from build123d import *

# Parameters (mm, degrees)
SKETCH1_R           = 25
BOSS_EXTRUDE1_DEPTH = 3
SKETCH2_R           = 1.75
CUT_EXTRUDE1_DEPTH  = 3
CIRPATTERN1_COUNT   = 8


with BuildPart() as part:
    # Sketch1 → Boss-Extrude1 (new body)
    with BuildSketch(Plane.XY):
        Circle(SKETCH1_R)
    extrude(amount=BOSS_EXTRUDE1_DEPTH)

    # Sketch2 → Cut-Extrude1 (cut)
    with BuildSketch(Plane.XY.offset(3)):
        with Locations((0, 20)):
            Circle(SKETCH2_R)
    cut_extrude1 = extrude(amount=-CUT_EXTRUDE1_DEPTH, mode=Mode.SUBTRACT)

    # CirPattern1: Cut-Extrude1 ×8 about axis
    cirpattern1_axis = Axis((0, 0, 0), (0, 0, 1))
    for i in range(1, CIRPATTERN1_COUNT):
        add(cut_extrude1.rotate(cirpattern1_axis, i * 360 / CIRPATTERN1_COUNT), mode=Mode.SUBTRACT)


solid = part.part
Model file for the job. Use its own axes, mm. Give positions to 0.01 mm unless a question says otherwise; leave off trailing zeros. Loops run counter-clockwise (first coordinate to the right, second up) from the corner with the lowest first, then second, coordinate; pieces in that order, holes last. Notation, with made-up numbers: (-18.75, 18.25) -> (-0.75, 18.25) arc R30 cw to (-0.75, 51.25) -> close; hole circle Ø11 at (86.25, 6.5). An arc over 180 degrees is marked (long way). Use a Markdown table: item, result. Add a question column.
(1) Wall check: line 1 along Y through (x, z) = (0, 2.2); line 2 along X through (y, z) = (-13, 0.1); line 3 along Y through (x, z) = (15, 0.35). Give the ranges that are in metal, low to high.
(2) Slice it at D-D on z = 0.8. Give the number of separate pieces and of enclosed holes in the cut face, and give its area (3 significant figures).
(3) Slice it at C-C on y = 0. List the corners of the cut face in (x, z).
(4) Mould opens along X. For faces 1 (the cylindrical face through (23.846, 7.509, 1.479)), 2 (the flat face through (0, 0, 3)), 3 (the cylindrical face through (12.525, -14.811, 1.521)) say: +X half, -X half, draft (parallel to the pull), parting line (faces both ways), or undercut.
(5) Drop flat-ended pins along their axis: pin 1 Ø3 at (x, y) = (14.14, 14.14) entering from +Z; pin 2 Ø1 at (y, z) = (-16.5, 2) entering from +X; pin 3 Ø1 at (x, y) = (15.5, -6) entering from -Z. Give the stop position or say it passes through.
(6) Slice it at A-A on y = 20. List the corners of the cut face in (x, z), and give its area (3 significant figures).
Filled sheet:
| question | item | result |
|---|---|---|
| 1 | line 1 | -25 to -21.75, -18.25 to 18.25, 21.75 to 25 |
| 1 | line 2 | -21.35 to -15.47, -12.82 to 12.82, 15.47 to 21.35 |
| 1 | line 3 | -20 to -15.67, -12.62 to 12.62, 15.67 to 20 |
| 2 | separate pieces | 1 |
| 2 | enclosed holes | 8 |
| 2 | area | 1,890 mm2 |
| 3 | outline | (-25, 0) -> (-21.75, 0) -> (-21.75, 3) -> (-25, 3) -> close; (-18.25, 0) -> (18.25, 0) -> (18.25, 3) -> (-18.25, 3) -> close; (21.75, 0) -> (25, 0) -> (25, 3) -> (21.75, 3) -> close |
| 4 | face 1 | parting line |
| 4 | face 2 | draft |
| 4 | face 3 | undercut |
| 5 | pin 1 | through |
| 5 | pin 2 | x = 19.21 |
| 5 | pin 3 | z = 0 |
| 6 | outline | (-15, 0) -> (-1.75, 0) -> (-1.75, 3) -> (-15, 3) -> close; (1.75, 0) -> (15, 0) -> (15, 3) -> (1.75, 3) -> close |
| 6 | area | 79.5 mm2 |
